from build123d import *

# Parameters (mm, degrees)
SKETCH_1_R          = 6.5
EXTRUDE_1_DEPTH     = 5
SKETCH_2_R          = 2
CUT_EXTRUDE_1_DEPTH = 6
SKETCH_3_R          = 5.6
SKETCH_3_R_2        = 3.35
CUT_EXTRUDE_2_DEPTH = 0.5
SKETCH_4_R          = 5.6
SKETCH_4_R_2        = 3.35
CUT_EXTRUDE_3_DEPTH = 0.5


with BuildPart() as part:
    # 草圖1 → 填料-伸長1 (new body)
    with BuildSketch(Plane.XY):
        Circle(SKETCH_1_R)
    extrude(amount=EXTRUDE_1_DEPTH)

    # 草圖2 → 除料-伸長1 (cut, through all)
    with BuildSketch(Plane.XY.offset(5)):
        Circle(SKETCH_2_R)
    extrude(amount=-CUT_EXTRUDE_1_DEPTH, mode=Mode.SUBTRACT)

    # 草圖3 → 除料-伸長2 (cut)
    with BuildSketch(Plane.XY.offset(5)):
        Circle(SKETCH_3_R)
        Circle(SKETCH_3_R_2, mode=Mode.SUBTRACT)
    extrude(amount=-CUT_EXTRUDE_2_DEPTH, mode=Mode.SUBTRACT)

    # 草圖4 → 除料-伸長3 (cut)
    with BuildSketch(Plane(origin=(0, 0, 0), x_dir=(-1, 0, 0), z_dir=(0, 0, -1))):
        Circle(SKETCH_4_R)
        Circle(SKETCH_4_R_2, mode=Mode.SUBTRACT)
    extrude(amount=-CUT_EXTRUDE_3_DEPTH, mode=Mode.SUBTRACT)


solid = part.part
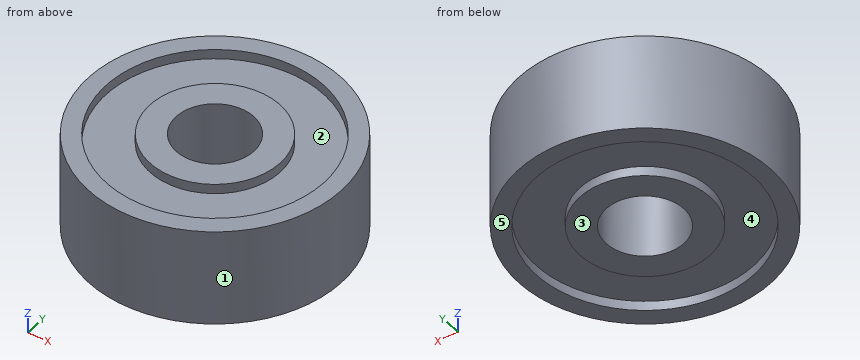
Can you work these out from the model? Positions are in its coordinate system, mm. Face numbers are marked on the shaded views. A direction names the side the tool comes from. Give positions to 0.01 mm unless a question says otherwise; leave off trailing zeros. Loops run counter-clockwise (first coordinate to the right, second up) from the corner with the lowest first, then second, coordinate; pieces in that order, holes last. Notation, with made-up numbers: (-2.5, 89) - (30.5, 89) arc R21 ccw to (30.5, 107) - close; hole circle Ø10 at (56, 29). An arc over 180 degrees is marked (long way). Return JSON: item names as keys, results as strings.
1. I want a section at C-C on z = 1.4. Please give me the cut outline in (x, y), and give its area (3 significant figures).
Output values:
{"outline": "circle Ø13 at (0, 0); hole circle Ø4 at (0, 0)", "area": "120 mm²"}
2. I want a section at D-D on y = 4. Please give me the cut outline in (x, z).
Output values:
{"outline": "(-5.12, 0) - (-3.92, 0) - (-3.92, 0.5) - (3.92, 0.5) - (3.92, 0) - (5.12, 0) - (5.12, 5) - (3.92, 5) - (3.92, 4.5) - (-3.92, 4.5) - (-3.92, 5) - (-5.12, 5) - close"}
3. I'm going to push flat-ended pins straight in: pin 1 Ø3.5 at (x, y) = (-1.5, 3) entering from -Z; pin 2 Ø3 at (y, z) = (-2, 1.5) entering from -X; pin 3 Ø1 at (y, z) = (3, 1) entering from +X; pin 4 Ø3 at (x, z) = (-2.5, 1) entering from +Y. Where does each tip first touch, or does it pass through?
Output values:
{"pin 1": "stops at z = 0", "pin 2": "stops at x = -6.48", "pin 3": "stops at x = 6", "pin 4": "stops at y = 6.42"}
4. I want a section at A-A on y = 0. Please give me the cut outline in (x, z), and give its area (3 significant figures).
Output values:
{"outline": "(-6.5, 0) - (-5.6, 0) - (-5.6, 0.5) - (-3.35, 0.5) - (-3.35, 0) - (-2, 0) - (-2, 5) - (-3.35, 5) - (-3.35, 4.5) - (-5.6, 4.5) - (-5.6, 5) - (-6.5, 5) - close; (2, 0) - (3.35, 0) - (3.35, 0.5) - (5.6, 0.5) - (5.6, 0) - (6.5, 0) - (6.5, 5) - (5.6, 5) - (5.6, 4.5) - (3.35, 4.5) - (3.35, 5) - (2, 5) - close", "area": "40.5 mm²"}
5. We'd pull the mould along X, two halves only. Please class the marked faces 1, 2 and 3: +X half, -X half, draft (parallel to the pull), parting line (faces both ways), or undercut.
Output values:
{"face 1": "parting line", "face 2": "undercut", "face 3": "draft"}
6. For the marked faces 4 and 5, which set-ups out of +Z, -Z, +X, -X, +Y, -Y let a thin tool reach every point of the face, with its end or its side?
Output values:
{"face 4": "-Z", "face 5": "-Z, +X, -X, +Y, -Y"}
7. If I drill on line 1 (Y direction, x = 0, z = 4.95); line 2 (Y direction, x = 0, z = 1.8); line 3 (Z direction, x = -5, y = 1), over which ranges is the centre line in solid material (lowest first)?
Output values:
{"line 1": "y = -6.5 to -5.6, -3.35 to -2, 2 to 3.35, 5.6 to 6.5", "line 2": "y = -6.5 to -2, 2 to 6.5", "line 3": "z = 0.5 to 4.5"}
